Model file for the job. Use its own axes, mm. Round coordinates to 2 decimals unless told otherwise and drop trailing zeros. Loops run counter-clockwise (first coordinate to the right, second up) from the corner with the lowest first, then second, coordinate; pieces in that order, holes last. Notation, with made-up numbers: (84, -9) -> (133, -9) arc R29 cw to (133, 20) -> close; hole circle Ø2 at (-4, -35). An arc over 180 degrees is marked (long way). Use a Markdown table: item, result.
from build123d import *

# Parameters (mm, degrees)
SKETCH1_R           = 73.025
BOSS_EXTRUDE1_DEPTH = 6.35


with BuildPart() as part:
    # Sketch1 → Boss-Extrude1 (new body)
    with BuildSketch(Plane(origin=(0, 0, 0), x_dir=(1, 0, 0), z_dir=(0, 1, 0))):
        with BuildLine():
            Line((79.44104, 6.985), (91.809669425, 6.985))
            ThreePointArc((91.809669425, 6.985), (65.106856878, 65.106856878), (6.985, 91.809669425))
            Line((6.985, 91.809669425), (6.985, 79.44104))
            Line((6.985, 79.44104), (-6.985, 79.44104))
            Line((-6.985, 79.44104), (-6.985, 91.809669425))
            ThreePointArc((-6.985, 91.809669425), (-65.106856878, 65.106856878), (-91.809669425, 6.985))
            Line((-91.809669425, 6.985), (-79.44104, 6.985))
            Line((-79.44104, 6.985), (-79.44104, -6.985))
            Line((-79.44104, -6.985), (-91.809669425, -6.985))
            ThreePointArc((-91.809669425, -6.985), (-65.106856878, -65.106856878), (-6.985, -91.809669425))
            Line((-6.985, -91.809669425), (-6.985, -79.44104))
            Line((-6.985, -79.44104), (6.985, -79.44104))
            Line((6.985, -79.44104), (6.985, -91.809669425))
            ThreePointArc((6.985, -91.809669425), (65.106856878, -65.106856878), (91.809669425, -6.985))
            Line((91.809669425, -6.985), (79.44104, -6.985))
            Line((79.44104, -6.985), (79.44104, 6.985))
        make_face()
        Circle(SKETCH1_R, mode=Mode.SUBTRACT)
    extrude(amount=BOSS_EXTRUDE1_DEPTH)


solid = part.part
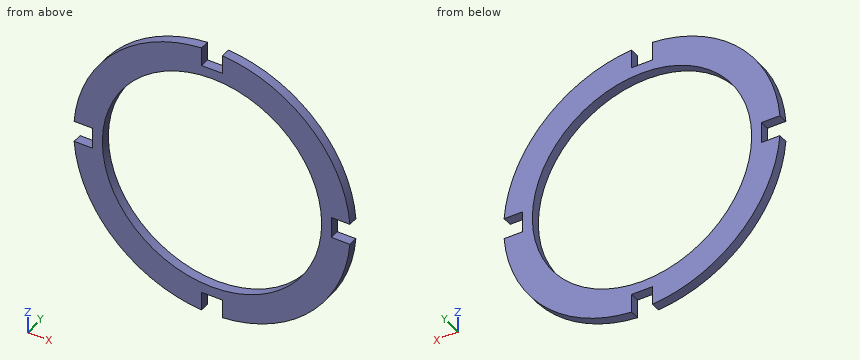
Q1. Flat gauge pins, fed straight in: pin 1 (1.9 mm diameter, centred on y = 3.5, z = -85, fed in from -X); pin 2 (1 mm diameter, centred on x = 69.5, y = 3, fed in from -Z); pin 3 (3 mm diameter, centred on x = 86.5, y = 4, fed in from -Z) (3 decimals). Where does each tip first touch, or does it go through?
Results list:
| item | result |
|---|---|
| pin 1 | stops at x = -37.6 |
| pin 2 | stops at z = -60.97 |
| pin 3 | stops at z = -35.395 |
Q2. Band-saw the part on A-A, the plane z = 0. Give the cut face in (x, y) (3 decimals).
Results list:
| item | result |
|---|---|
| outline | (-79.441, 0) -> (-73.025, 0) -> (-73.025, 6.35) -> (-79.441, 6.35) -> close; (73.025, 0) -> (79.441, 0) -> (79.441, 6.35) -> (73.025, 6.35) -> close |
Q3. Band-saw the part on C-C, the plane y = 3.75. Give the cut face in (x, z) (3 decimals), plus the area to 3 significant figures.
Results list:
| item | result |
|---|---|
| outline | (-91.81, -6.985) arc R92.075 ccw to (-6.985, -91.81) -> (-6.985, -79.441) -> (6.985, -79.441) -> (6.985, -91.81) arc R92.075 ccw to (91.81, -6.985) -> (79.441, -6.985) -> (79.441, 6.985) -> (91.81, 6.985) arc R92.075 ccw to (6.985, 91.81) -> (6.985, 79.441) -> (-6.985, 79.441) -> (-6.985, 91.81) arc R92.075 ccw to (-91.81, 6.985) -> (-79.441, 6.985) -> (-79.441, -6.985) -> close; hole circle Ø146.05 at (0, 0) |
| area | 9,180 mm² |
Q4. Band-saw the part on B-B, the plane x = 48.5. Give the cut face in (y, z).
Results list:
| item | result |
|---|---|
| outline | (0, -78.27) -> (6.35, -78.27) -> (6.35, -54.59) -> (0, -54.59) -> close; (0, 54.59) -> (6.35, 54.59) -> (6.35, 78.27) -> (0, 78.27) -> close |
Q5. Drill centre lines: L1, parallel to X at y = 2, z = 0 (3 decimals); L2, parallel to Z at x = 51.5, y = 4. Where is each one in solid material? Low to high. Write a range as from..to.
Results list:
| item | result |
|---|---|
| L1 | x = -79.441..-73.025, 73.025..79.441 |
| L2 | z = -76.33..-51.77, 51.77..76.33 |
